Part model, mm, in its own coordinate system. A direction names the side the tool comes from. Round coordinates to 2 decimals unless told otherwise and drop trailing zeros. Order: outer loops, then holes, each group sorted by start corner. A loop starts at its lowest first (then second) coordinate and runs counter-clockwise, first axis right, second up. Notation, with made-up numbers: (-35, 34.5) - (23, 34.5) arc R17 ccw to (23, 62.5) - close; hole circle Ø6 at (14.25, 74.25). An arc over 180 degrees is marked (long way). Answer as a JSON object with one key per item and string values.
Autodesk Inventor part; units mm, degrees
ref_plane "YZ Plane" through (0, 0, 0) normal (1, 0, 0) x (0, 1, 0)
ref_plane "XZ Plane" through (0, 0, 0) normal (0, 1, 0) x (-1, 0, 0)
ref_plane "XY Plane" through (0, 0, 0) normal (0, 0, 1) x (1, 0, 0)
sketch "Sketch1" plane through (0, 0, 0) normal (0, 1, 0) x (-1, 0, 0)
  arc A0 (38.1, 33.601) -> (-38.1, 33.601) centre (0, 0) ccw
  line L0 (38.1, -33.601) -> (38.1, 33.601)
  arc A1 (38.1, -33.601) -> (38.1, 33.601) centre (0, 0) ccw construction
  line L1 (-38.1, -33.601) -> (-38.1, 33.601)
  arc A2 (-38.1, -33.601) -> (38.1, -33.601) centre (0, 0) ccw
  arc A3 (-38.1, 33.601) -> (-38.1, -33.601) centre (0, 0) ccw construction
  dimension "d0" = 101.6
  dimension "d3" = 12.7
  dimension "d4" = 76.2
extrude "Extrusion1" add sketch "Sketch1" along normal blind 3.175
sketch "Sketch2" plane through (0, 3.175, 0) normal (0, 1, 0) x (1, 0, 0)
  line L0 (-38.1, 33.601) -> (38.1, 33.601) construction
  line L1 (38.1, -33.601) -> (-38.1, -33.601) construction
  line L2 (-38.1, -6.0865) -> (38.1, -6.0865) construction
  line L3 (38.1, 33.601) -> (38.1, -33.601) construction
  line L4 (38.1, -33.601) -> (38.1, 33.601) construction
  line L5 (-19.05, 27.251) -> (19.05, 27.251)
  line L6 (19.05, 24.076) -> (-19.05, 24.076)
  arc A0 (-19.05, 27.251) -> (-19.05, 24.076) centre (-19.05, 25.6635) ccw
  arc A1 (19.05, 24.076) -> (19.05, 27.251) centre (19.05, 25.6635) ccw
  line L7 (-38.1, 33.601) -> (-38.1, -33.601)
  line L8 (-19.05, -39.424) -> (19.05, -39.424)
  line L9 (19.05, -36.249) -> (-19.05, -36.249)
  arc A2 (-19.05, -36.249) -> (-19.05, -39.424) centre (-19.05, -37.8365) ccw
  arc A3 (19.05, -39.424) -> (19.05, -36.249) centre (19.05, -37.8365) ccw
  point P0 (0, 0)
  dimension "d11" = 19.05
  dimension "d12" = 19.05
  dimension "d13" = 6.35
  dimension "d14" = 3.175
  dimension "d17" = 63.5
extrude "Extrusion2" cut sketch "Sketch2" against normal through all
properties part number "top"
Item 1: Cut at A-A (x = -0.5). Write the cut outline in (y, z) (3 decimals).
Taken from the geometry:
{"outline": "(0, -50.798) - (3.175, -50.798) - (3.175, -27.251) - (0, -27.251) - close; (0, -24.076) - (3.175, -24.076) - (3.175, 36.249) - (0, 36.249) - close; (0, 39.424) - (3.175, 39.424) - (3.175, 50.798) - (0, 50.798) - close"}
Item 2: Probe L1, parallel to Z at x = 17, y = 2.8; L2, parallel to Z at x = -8, y = 1.9; L3, parallel to X at y = 0.15, z = 37.5. List the from-to ranges inside material, lowest first. Write a range as from..to.
Taken from the geometry:
{"L1": "-47.87..-27.25, -24.08..36.25, 39.42..47.87", "L2": "-50.17..-27.25, -24.08..36.25, 39.42..50.17", "L3": "-34.27..-20.6, 20.6..34.27"}
Item 3: Cut at D-D (x = 26.5). Write the cut outline in (y, z) (3 decimals), plus the area to 3 significant figures.
Taken from the geometry:
{"outline": "(0, -43.34) - (3.175, -43.34) - (3.175, 43.34) - (0, 43.34) - close", "area": "275 mm2"}
Item 4: Tool access for faces 4 (the flat face through (0, 2, -24.076)), 5 (the flat face through (1, 0, 1)): list every direction of +Z, -Z, +X, -X, +Y, -Y with a clear straight run to the whole face (end or side of a thin tool).
Taken from the geometry:
{"face 4": "+Y, -Y", "face 5": "+Z, -Z, +X, -X, -Y"}
Item 5: Cut at B-B (y = 2.05). State how many separate pieces and enclosed holes the cut face has, plus the area to 3 significant figures.
Taken from the geometry:
{"separate pieces": "1", "enclosed holes": "2", "area": "6,680 mm2"}
Item 6: Cut at C-C (x = 9). Write the cut outline in (y, z) (3 decimals).
Taken from the geometry:
{"outline": "(0, -49.996) - (3.175, -49.996) - (3.175, -27.251) - (0, -27.251) - close; (0, -24.076) - (3.175, -24.076) - (3.175, 36.249) - (0, 36.249) - close; (0, 39.424) - (3.175, 39.424) - (3.175, 49.996) - (0, 49.996) - close"}
Item 7: Two-plate mould, pull along X, no slides. Class faces 1 (the cylindrical face through (-0.603, 1.565, -50.796)), 2 (the flat face through (38.1, 2, 0)), 3 (the cylindrical face through (-20.637, 1.61, 37.802)): pulls with the +X half, pulls with the -X half, needs draft (parallel to the pull), parting line crosses it, or undercut.
Taken from the geometry:
{"face 1": "parting line crosses it", "face 2": "pulls with the +X half", "face 3": "undercut"}
Item 8: Drop flat-ended pins along their axis: P1, Ø10, axis at x = 25.5, z = 5.5, coming from the -Y side; P2, Ø1.6, axis at x = -3, y = 1.5, coming from the -Z side; P3, Ø1.5, axis at x = 30.5, y = 1.5, coming from the -Z side; P4, Ø1.6, axis at x = 9.5, y = 2.5, coming from the +Z side. Give the stop position or say it passes through.
Taken from the geometry:
{"P1": "y = 0", "P2": "z = -50.75", "P3": "z = -41.18", "P4": "z = 50.05"}
